```python
from build123d import *

# Parameters (mm, degrees)
F0_W     = 88.9
F0_H     = 127
F1_DEPTH = 63.5
F2_W     = 38.1
F2_H     = 63.5
F3_DEPTH = 15.24
F5_DEPTH = 31.75


with BuildPart() as f1:
    # F0 (on Top) → F1 (new body)
    with BuildSketch(Plane.XY):
        with Locations((-0.36866225, 6.5260546505)):
            Rectangle(F0_W, F0_H)
    extrude(amount=F1_DEPTH)

    # F2 (on face) → F3 (cut)
    with BuildSketch(Plane.XY.offset(63.5)):
        with Locations((25.03133775, 38.2760546505)):
            Rectangle(F2_W, F2_H)
    extrude(amount=-F3_DEPTH, mode=Mode.SUBTRACT)

    # F4 (on face) → F5 (cut)
    with BuildSketch(Plane.XY.offset(63.5)):
        Polygon((44.08133775, 6.5260546505), (5.98133775, 6.5260546505), (-44.81866225, 6.5260546505), (-44.81866225, -56.9739453495), (44.08133775, -56.9739453495), align=None)
    extrude(amount=-F5_DEPTH, mode=Mode.SUBTRACT)


solid = f1.part
```
Model file for the job. Use its own axes, mm. A direction names the side the tool comes from. Round coordinates to 2 decimals unless told otherwise and drop trailing zeros. Write each loop counter-clockwise with the first axis right and the second up, starting at its lowest first coordinate (ties: lowest second). Pieces come first, ordered by that corner, then holes. Notation, with made-up numbers: M 30.5,6 L 67.5,6 A20 ccw 67.5,10 Z; hole C 57.25,-30.75 d1. An arc over 180 degrees is marked long. Put each result on its own line as item: value.
Item 1: Cut at B-B (x = 27). List the corners of the cut face in (y, z).
Responses:
outline: M -56.97,0 L 70.03,0 L 70.03,48.26 L 6.53,48.26 L 6.53,31.75 L -56.97,31.75 Z
Item 2: Tool access for faces 1 (the flat face through (-1, -25, 31.75)), 2 (the flat face through (5.981, 38, 56)), 3 (the flat face through (-1, -56.974, 16)): list every direction of +Z, -Z, +X, -X, +Y, -Y with a clear straight run to the whole face (end or side of a thin tool).
Responses:
face 1: +Z, +X, -X, -Y
face 2: +Z, +X, +Y, -Y
face 3: +Z, -Z, +X, -X, -Y
Item 3: Cut at D-D (z = 56). List the corners of the cut face in (x, y).
Responses:
outline: M -44.82,6.53 L 5.98,6.53 L 5.98,70.03 L -44.82,70.03 Z
Item 4: Cut at A-A (y = 31). List the corners of the cut face in (x, z).
Responses:
outline: M -44.82,0 L 44.08,0 L 44.08,48.26 L 5.98,48.26 L 5.98,63.5 L -44.82,63.5 Z
Item 5: Probe L1, parallel to X at y = 36.5, z = 54; L2, parallel to Z at x = 21, y = 32; L3, parallel to Z at x = 39, y = -26. List the from-to ranges inside material, lowest first. Write a range as from..to.
Responses:
L1: -44.82..5.98
L2: 0..48.26
L3: 0..31.75
Item 6: Flat gauge pins, fed straight in: P1, Ø9.5, axis at x = -20.5, z = 48, coming from the -Y side; P2, Ø12, axis at y = 46.5, z = 57.5, coming from the +X side; P3, Ø19, axis at x = 27.5, y = 35.5, coming from the +Z side. Where does each tip first touch, or does it go through?
Responses:
P1: y = 6.53
P2: x = 5.98
P3: z = 48.26
Item 7: Cut at C-C (z = 36.5). List the corners of the cut face in (x, y).
Responses:
outline: M -44.82,6.53 L 44.08,6.53 L 44.08,70.03 L -44.82,70.03 Z
